Build history of the part. All positions in model axes, mm. A direction names the side the tool comes from. Round coordinates to 2 decimals unless told otherwise and drop trailing zeros. Loops run counter-clockwise (first coordinate to the right, second up) from the corner with the lowest first, then second, coordinate; pieces in that order, holes last. Notation, with made-up numbers: (-11.75, 88.25) - (45.25, 88.25) arc R29 cw to (45.25, 122.25) - close; hole circle Ø4 at (-11.5, -38.5). An arc over 180 degrees is marked (long way). Use a Markdown table: item, result.
from build123d import *

# Parameters (mm, degrees)
BOSS_EXTRUDE2_DEPTH = 4
FILLET1_R           = 4
SKETCH6_R           = 1.5
CUT_EXTRUDE1_DEPTH  = 4
SKETCH3_R           = 1.5
CUT_EXTRUDE2_DEPTH  = 4
SKETCH7_W           = 3.00651588
SKETCH7_H           = 15.442
BOSS_EXTRUDE3_DEPTH = 35
FILLET2_R           = 3
FILLET3_R           = 3


with BuildPart() as part:
    # Sketch2 → Boss-Extrude2 (new body)
    with BuildSketch(Plane.XY):
        Polygon((-67.081093968, -2.634474623), (-67.081093968, 16.923525377), (-26.695093968, 16.923525377), (-26.695093968, -2.634474623), (-19.075093968, -2.634474623), (-19.075093968, 32.365525377), (-67.081093968, 32.365525377), (-74.701093968, 32.365525377), (-156.39106061, 32.365525377), (-156.39106061, 16.923525377), (-74.701093968, 16.923525377), (-74.701093968, -2.634474623), align=None)
    extrude(amount=BOSS_EXTRUDE2_DEPTH)

    # Fillet1
    fillet1_edges = [part.edges().sort_by_distance(p)[0] for p in [
        (-19.075093968, 32.365525377, 2),
        (-19.075093968, -2.634474623, 2),
        (-74.701093968, -2.634474623, 2),
    ]]
    fillet(fillet1_edges, radius=FILLET1_R)

    # Sketch6 → Cut-Extrude1 (cut)
    with BuildSketch(Plane.XY.offset(4)):
        with Locations((-71.018093968, 12.224525377)):
            Circle(SKETCH6_R)
        with Locations((-22.758093968, 12.224525377)):
            Circle(SKETCH6_R)
        with Locations((-22.758093968, 2.064525377)):
            Circle(SKETCH6_R)
        with Locations((-71.018093968, 2.064525377)):
            Circle(SKETCH6_R)
    extrude(amount=-CUT_EXTRUDE1_DEPTH, mode=Mode.SUBTRACT)

    # Sketch3 → Cut-Extrude2 (cut)
    with BuildSketch(Plane.XY.offset(4)):
        with Locations((-145.701093968, 25.365525377)):
            Circle(SKETCH3_R)
        with Locations((-88.701093968, 25.365525377)):
            Circle(SKETCH3_R)
    extrude(amount=-CUT_EXTRUDE2_DEPTH, mode=Mode.SUBTRACT)

    # Sketch7 → Boss-Extrude3 (add)
    with BuildSketch(Plane.XY.offset(4)):
        with Locations((-154.88780267, 24.644525377)):
            Rectangle(SKETCH7_W, SKETCH7_H)
    extrude(amount=BOSS_EXTRUDE3_DEPTH)

    # Fillet2
    fillet2_edges = [part.edges().sort_by_distance(p)[0] for p in [
        (-153.38454473, 24.644525377, 4),
    ]]
    fillet(fillet2_edges, radius=FILLET2_R)

    # Fillet3
    fillet3_edges = [part.edges().sort_by_distance(p)[0] for p in [
        (-156.39106061, 24.644525377, 0),
    ]]
    fillet(fillet3_edges, radius=FILLET3_R)


solid = part.part
Q1. Probe line 1 (X direction, y = 23, z = 9); line 2 (Z direction, x = -65.5, y = 18). List the from-to ranges inside material, lowest first.
Results found:
| item | result |
|---|---|
| line 1 | x = -156.39 to -153.38 |
| line 2 | z = 0 to 4 |
Q2. Cut at A-A, the plane y = 6.5. List the corners of the cut face in (x, z), plus the area to 3 significant figures.
Results found:
| item | result |
|---|---|
| outline | (-74.7, 0) - (-67.08, 0) - (-67.08, 4) - (-74.7, 4) - close; (-26.7, 0) - (-19.08, 0) - (-19.08, 4) - (-26.7, 4) - close |
| area | 61.0 mm2 |
Q3. Cut at D-D, the plane x = -54.5. List the corners of the cut face in (y, z).
Results found:
| item | result |
|---|---|
| outline | (16.92, 0) - (32.37, 0) - (32.37, 4) - (16.92, 4) - close |
Q4. Drop flat-ended pins along their axis: pin 1 (10.5 mm diameter, centred on x = -110, y = 15.5, fed in from +Z); pin 2 (3 mm diameter, centred on y = 15.5, z = 17.5, fed in from +X); pin 3 (1.2 mm diameter, centred on y = 10, z = 1, fed in from -X). Give the stop position or say it passes through.
Results found:
| item | result |
|---|---|
| pin 1 | stops at z = 4 |
| pin 2 | stops at x = -153.38 |
| pin 3 | stops at x = -74.7 |
Q5. Which spindle directions (+Z, -Z, +X, -X, +Y, -Y) get a long thin tool onto all of the face, cutting with end or side? Do faces 5 (the face through (-124.8, 16.924, 3.5)), 6 (the face through (-155, 25, 39)), 7 (the face through (-47, 16.924, 2)), 8 (the face through (-153.385, 25, 23)), 9 (the face through (-104.9, 32.366, 3.5)). Say none if no direction does.
Results found:
| item | result |
|---|---|
| face 5 | +Z, -Z, -X, -Y |
| face 6 | +Z, +X, -X, +Y, -Y |
| face 7 | +Z, -Z, -Y |
| face 8 | +Z, +X, +Y, -Y |
| face 9 | +Z, -Z, +X, -X, +Y |
Q6. Cut at C-C, the plane z = 12. List the corners of the cut face in (x, y), plus the area to 3 significant figures.
Results found:
| item | result |
|---|---|
| outline | (-156.39, 16.92) - (-153.38, 16.92) - (-153.38, 32.37) - (-156.39, 32.37) - close |
| area | 46.4 mm2 |
Q7. Cut at B-B, the plane y = 21. List the corners of the cut face in (x, z).
Results found:
| item | result |
|---|---|
| outline | (-156.39, 3) arc R3 ccw to (-153.39, 0) - (-19.08, 0) - (-19.08, 4) - (-150.38, 4) arc R3 cw to (-153.38, 7) - (-153.38, 39) - (-156.39, 39) - close |
Q8. Pull direction Y, two halves, no side cores. Call faces 1 (the face through (-69, -2.634, 2)), 2 (the face through (-19.075, 15, 2)), 3 (the face through (-72.517, 12.29, 2.028)), 4 (the face through (-20.216, 31.163, 2.028)): pulls with the +Y half, pulls with the -Y half, needs draft (parallel to the pull), parting line crosses it, or undercut.
Results found:
| item | result |
|---|---|
| face 1 | pulls with the -Y half |
| face 2 | needs draft |
| face 3 | undercut |
| face 4 | pulls with the +Y half |
